Input: part model. Units: mm. Frame: model coordinates. A direction names the side the tool comes from. Coordinates: 2 decimals unless noted, no trailing zeros. Loops run counter-clockwise (first coordinate to the right, second up) from the corner with the lowest first, then second, coordinate; pieces in that order, holes last. Notation, with made-up numbers: (-24.75, 63.25) -> (-18.75, 63.25) arc R14 cw to (-18.75, 79.25) -> close; hole circle Ø2 at (45, 58.5). An arc over 180 degrees is marked (long way). Answer as a JSON object with one key per item and string values.
from build123d import *

# Parameters (mm, degrees)
F0_W          = 100
F0_H          = 100
F1_DEPTH      = 4
F2_W          = 100
F2_H          = 8
F3_DEPTH      = 20
F5_DEPTH      = 58.001
F5_DEPTH_BACK = 58.001


with BuildPart() as f1:
    # F0 (on Top) → F1 (new body)
    with BuildSketch(Plane.XY):
        Rectangle(F0_W, F0_H)
        with BuildLine():
            Line((3.5, 32.5), (3.5, -32.5))
            ThreePointArc((3.5, -32.5), (0, -36), (-3.5, -32.5))
            Line((-3.5, -32.5), (-3.5, 32.5))
            ThreePointArc((-3.5, 32.5), (0, 36), (3.5, 32.5))
        make_face(mode=Mode.SUBTRACT)
    extrude(amount=F1_DEPTH)

    # F2 (on Top) → F3 (join)
    with BuildSketch(Plane.XY):
        with Locations((0, 54)):
            Rectangle(F2_W, F2_H)
        with Locations((0, -54)):
            Rectangle(F2_W, F2_H)
    extrude(amount=F3_DEPTH)

    # F4 (on Front) → F5 (cut, two sides)
    with BuildSketch(Plane.XZ) as f5_sk:
        with BuildLine():
            ThreePointArc((-38.6532023549, 15), (-41.6532023549, 12), (-38.6532023549, 9))
            Line((-38.6532023549, 9), (43.4487722814, 9))
            ThreePointArc((43.4487722814, 9), (46.4487722814, 12), (43.4487722814, 15))
            Line((43.4487722814, 15), (-38.6532023549, 15))
        make_face()
    extrude(amount=-F5_DEPTH, mode=Mode.SUBTRACT)
    extrude(f5_sk.sketch, amount=F5_DEPTH_BACK, mode=Mode.SUBTRACT)


solid = f1.part
1. Line query: line 1 along Y through (x, z) = (-46, 11.75); line 2 along X through (y, z) = (-18.5, 3.5); line 3 along Z through (x, y) = (31, 44.5). Output: solid intervals per line, ascending.
Reply:
{"line 1": "y = -58 to -50, 50 to 58", "line 2": "x = -50 to -3.5, 3.5 to 50", "line 3": "z = 0 to 4"}
2. Section query C-C (y = 29). Return loops of the section in (x, z), plus the area to 3 significant figures.
Reply:
{"outline": "(-50, 0) -> (-3.5, 0) -> (-3.5, 4) -> (-50, 4) -> close; (3.5, 0) -> (50, 0) -> (50, 4) -> (3.5, 4) -> close", "area": "372 mm2"}
3. Access query for faces 4 (the face through (3.5, 0, 2)), 5 (the face through (-41.652, -53.944, 12.066)), 6 (the face through (50, -1, 3)), 7 (the face through (10, 1, 4)). Directions: +Z, -Z, +X, -X, +Y, -Y. A direction counts if a zero-diameter tool reaches every point of the face in a straight line with its end or side. Return the directions, or none.
Reply:
{"face 4": "+Z, -Z", "face 5": "+Y, -Y", "face 6": "+Z, -Z, +X, +Y, -Y", "face 7": "+Z, +X, -X"}
4. Section query B-B (z = 12). Return loops of the section in (x, y), plus the area to 3 significant figures.
Reply:
{"outline": "(-50, -58) -> (-41.65, -58) -> (-41.65, -50) -> (-50, -50) -> close; (-50, 50) -> (-41.65, 50) -> (-41.65, 58) -> (-50, 58) -> close; (46.45, -58) -> (50, -58) -> (50, -50) -> (46.45, -50) -> close; (46.45, 50) -> (50, 50) -> (50, 58) -> (46.45, 58) -> close", "area": "190 mm2"}
5. Section query D-D (x = 25). Return loops of the section in (y, z).
Reply:
{"outline": "(-58, 0) -> (58, 0) -> (58, 9) -> (50, 9) -> (50, 4) -> (-50, 4) -> (-50, 9) -> (-58, 9) -> close; (-58, 15) -> (-50, 15) -> (-50, 20) -> (-58, 20) -> close; (50, 15) -> (58, 15) -> (58, 20) -> (50, 20) -> close"}
6. Section query A-A (x = 0). Return loops of the section in (y, z).
Reply:
{"outline": "(-58, 0) -> (-36, 0) -> (-36, 4) -> (-50, 4) -> (-50, 9) -> (-58, 9) -> close; (-58, 15) -> (-50, 15) -> (-50, 20) -> (-58, 20) -> close; (36, 0) -> (58, 0) -> (58, 9) -> (50, 9) -> (50, 4) -> (36, 4) -> close; (50, 15) -> (58, 15) -> (58, 20) -> (50, 20) -> close"}
7. Mould query, pull axis X, two halves, no side actions, for faces 1 (the face through (-50, -1, 3)), 2 (the face through (-1, 58, 8)), 3 (the face through (46.448, -53.944, 11.934)). Classes: pulls with the +X half, pulls with the -X half, needs draft (parallel to the pull), parting line crosses it, or undercut.
Reply:
{"face 1": "pulls with the -X half", "face 2": "needs draft", "face 3": "undercut"}
8. Pin query (flat end, axial travel): P1, Ø4, axis at x = 3, y = 18, coming from the +Z side. Return the tip coordinate at first contact, or that it passes through.
Reply:
{"P1": "stops at z = 4"}
